from build123d import *

# Parameters (mm, degrees)
F0_W           = 50.8
F0_H           = 50.8
F1_DEPTH       = 19.05
F4_R           = 15.875
F3_R           = 9.525
F7_D           = 4.9784
F7_CSINK_D     = 10.4394
F7_CSINK_ANGLE = 82
F8_R           = 2.794
F8_R_2         = 2.286
F9_DEPTH       = 15.875


with BuildPart() as f1:
    # F0 (on Top) → F1 (new body)
    with BuildSketch(Plane.XY):
        Rectangle(F0_W, F0_H)
    extrude(amount=F1_DEPTH)

    # F4 (on face) → F5 section 0
    with BuildSketch(Plane.XY.offset(19.05)):
        Circle(F4_R)
    # F3 (on offset) → F5 section 1
    with BuildSketch(Plane.XY.offset(50.8)):
        Circle(F3_R)
    loft()

    # F7 (through all)
    with Locations(Plane.XY.offset(19.05)):
        with Locations((-19.05, 19.05), (19.05, 19.05), (19.05, -19.05), (-19.05, -19.05)):
            CounterSinkHole(F7_D / 2, F7_CSINK_D / 2, counter_sink_angle=F7_CSINK_ANGLE)

    # F8 (on face) → F9 (join)
    with BuildSketch(Plane(origin=(0, 0, 0), x_dir=(1, 0, 0), z_dir=(0, 0, -1))):
        with Locations((19.05, -19.05)):
            Circle(F8_R)
        with Locations((19.05, -19.05)):
            Circle(F8_R_2, mode=Mode.SUBTRACT)
        with Locations((19.05, 19.05)):
            Circle(F8_R)
        with Locations((19.05, 19.05)):
            Circle(F8_R_2, mode=Mode.SUBTRACT)
        with Locations((-19.05, 19.05)):
            Circle(F8_R)
        with Locations((-19.05, 19.05)):
            Circle(F8_R_2, mode=Mode.SUBTRACT)
        with Locations((-19.05, -19.05)):
            Circle(F8_R)
        with Locations((-19.05, -19.05)):
            Circle(F8_R_2, mode=Mode.SUBTRACT)
    extrude(amount=-F9_DEPTH)


solid = f1.part
Can you work these out from the model? Positions are in its coordinate system, mm. Give positions to 0.01 mm unless a question says otherwise; leave off trailing zeros. Order: outer loops, then holes, each group sorted by start corner. A loop starts at its lowest first (then second) coordinate and runs counter-clockwise, first axis right, second up. Notation, with made-up numbers: (36.25, 69) - (75.25, 69) arc R14 ccw to (75.25, 96) - close; hole circle Ø1 at (55, 2). An arc over 180 degrees is marked (long way). Write each question's results on one line, items separated by ' | '.
1) I'm going to push flat-ended pins straight in: pin 1 Ø3 at (x, y) = (11.5, -18.5) entering from +Z; pin 2 Ø1.5 at (x, z) = (-5, 38.5) entering from +Y; pin 3 Ø4 at (x, y) = (19, 18) entering from +Z; pin 4 Ø10 at (x, y) = (-12, 5) entering from -Z. Where does each tip first touch, or does it pass through?
Final values:
pin 1: stops at z = 19.05 | pin 2: stops at y = 11.25 | pin 3: stops at z = 16.56 | pin 4: stops at z = 0
2) Suppose I cut it at D-D, the plane x = 0. Write out the boundary of the cut face in (y, z) (3 decimals), then the cut area to 3 significant figures.
Final values:
outline: (-25.4, 0) - (25.4, 0) - (25.4, 19.05) - (15.875, 19.05) - (9.525, 50.8) - (-9.525, 50.8) - (-15.875, 19.05) - (-25.4, 19.05) - close | area: 1,770 mm^2
3) If we mould it in two halves opening along Y, with no side actions, what happens to faces 1 (the face through (-25.4, 0, 9)), 2 (the face through (-18.71, -16.45, 16.06)), 3 (the face through (-2.591, -11.666, 38.675)), 4 (the face through (0, -25.4, 9))? For each: pulls with the +Y half, pulls with the -Y half, needs draft (parallel to the pull), parting line crosses it, or undercut.
Final values:
face 1: needs draft | face 2: undercut | face 3: parting line crosses it | face 4: pulls with the -Y half
4) Suppose I cut it at A-A, the plane z = 14. Write out the boundary of the cut face in (x, y).
Final values:
outline: (-25.4, -25.4) - (25.4, -25.4) - (25.4, 25.4) - (-25.4, 25.4) - close; hole circle Ø4.57 at (-19.05, -19.05); hole circle Ø4.57 at (-19.05, 19.05); hole circle Ø4.57 at (19.05, -19.05); hole circle Ø4.57 at (19.05, 19.05)
5) Please list where these lines run through material, in increasing order: line 1 along Y through (x, z) = (-19.05, 10.75); line 2 along Y through (x, z) = (-19.05, 15.95). Write a range as [from, to].
Final values:
line 1: y = [-25.4, -21.34], [-16.76, 16.76], [21.34, 25.4] | line 2: y = [-25.4, -21.57], [-16.53, 16.53], [21.57, 25.4]
6) Suppose I cut it at B-B, the plane y = -19.05. Write out the boundary of the cut face in (x, z) (3 decimals), then the cut area to 3 significant figures.
Final values:
outline: (-25.4, 0) - (-21.336, 0) - (-21.336, 15.875) - (-21.539, 15.875) - (-21.539, 15.909) - (-24.27, 19.05) - (-25.4, 19.05) - close; (-16.764, 0) - (16.764, 0) - (16.764, 15.875) - (16.561, 15.875) - (16.561, 15.909) - (13.83, 19.05) - (-13.83, 19.05) - (-16.561, 15.909) - (-16.561, 15.875) - (-16.764, 15.875) - close; (21.336, 0) - (25.4, 0) - (25.4, 19.05) - (24.27, 19.05) - (21.539, 15.909) - (21.539, 15.875) - (21.336, 15.875) - close | area: 774 mm^2
